The model under review builds one solid part; all positions refer to its coordinate system, in mm. Face numbers are marked on the shaded views. A direction names the side the tool comes from. Round coordinates to 2 decimals unless told otherwise and drop trailing zeros. Loops run counter-clockwise (first coordinate to the right, second up) from the corner with the lowest first, then second, coordinate; pieces in that order, holes last. Notation, with made-up numbers: M 75.5,18 L 115.5,18 A26 ccw 115.5,34 Z; hole C 42,15 d8. An arc over 180 degrees is marked long. Answer as a JSON object with one key per item and string values. Group by question number.
Item 1: Consider section B-B (x = 31.5). Give the boundary of the cut face in (y, z).
Item 2: Tool access review of the marked faces 1 and 2: name each direction out of +Z, -Z, +X, -X, +Y, -Y from which nothing blocks a thin tool from reaching the whole face with its end or side.
Item 3: Consider section A-A (z = 9). Give the boundary of the cut face in (x, y).
Item 4: To check wall thickness, follow line 1 (Z direction, x = 39, y = 28.5); line 2 (Y direction, x = 55.5, z = 7); line 3 (X direction, y = 26.5, z = 13). State the ranges of each line that lie inside material, in increasing order.
Item 5: Insertion check: P1, Ø4.5, axis at y = 27.5, z = 5.5, coming from the +X side; P2, Ø4.5, axis at x = 53.5, z = 8.5, coming from the +Y side; P3, Ø9, axis at x = 57, y = 36, coming from the -Z side. Each pin has a flat end and moves straight along its axis. Give the tip position at first contact, or say it passes through.
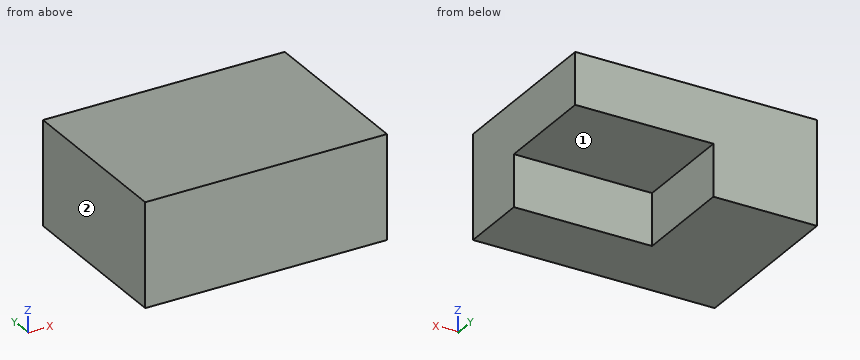
```python
from build123d import *

# Parameters (mm, degrees)
BOSS_EXTRUDE3_DEPTH      = 30
BOSS_EXTRUDE3_DEPTH_BACK = 0.0001
SKETCH4_W                = 70
SKETCH4_H                = 20
SKETCH6_W                = 30
SKETCH6_H                = 30.0001
BOSS_EXTRUDE4_DEPTH      = 30
SKETCH7_W                = 40
SKETCH7_H                = 15.00005
BOSS_EXTRUDE5_DEPTH      = 30


with BuildPart() as part:
    # Sketch4 → Boss-Extrude3 (new, two sides: drawn at the far end of the back side and taken through both)
    with BuildSketch(Plane.XY.offset(-BOSS_EXTRUDE3_DEPTH_BACK)):
        with Locations((35, 10)):
            Rectangle(SKETCH4_W, SKETCH4_H)
    extrude(amount=BOSS_EXTRUDE3_DEPTH + BOSS_EXTRUDE3_DEPTH_BACK)

    # Sketch6 → Boss-Extrude4 (add)
    with BuildSketch(Plane(origin=(0, 20, 0), x_dir=(1, 0, 0), z_dir=(0, 1, 0))):
        with Locations((15, -14.99995)):
            Rectangle(SKETCH6_W, SKETCH6_H)
    extrude(amount=BOSS_EXTRUDE4_DEPTH)

    # Sketch7 → Boss-Extrude5 (add)
    with BuildSketch(Plane(origin=(0, 20, 0), x_dir=(1, 0, 0), z_dir=(0, 1, 0))):
        with Locations((50, -22.499975)):
            Rectangle(SKETCH7_W, SKETCH7_H)
    extrude(amount=BOSS_EXTRUDE5_DEPTH)


solid = part.part
```
Geometry results:
{
 "1": {"outline": "M 0,0 L 20,0 L 20,15 L 50,15 L 50,30 L 0,30 Z"},
 "2": {"face 1": "-Z, +X, +Y", "face 2": "+Z, -Z, -X, +Y, -Y"},
 "3": {"outline": "M 0,0 L 70,0 L 70,20 L 30,20 L 30,50 L 0,50 Z"},
 "4": {"line 1": "z = 15 to 30", "line 2": "y = 0 to 20", "line 3": "x = 0 to 30"},
 "5": {"P1": "stops at x = 30", "P2": "stops at y = 20", "P3": "stops at z = 15"}
}
